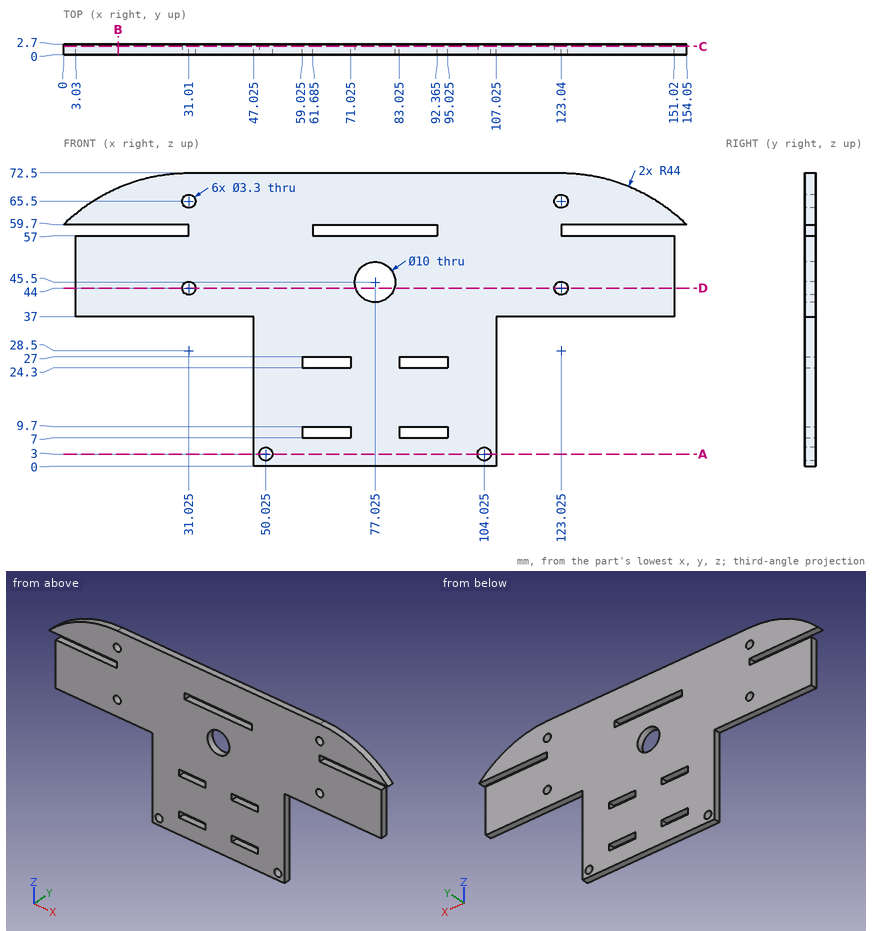
Check sheet for the drawn part. Datum: minimum x, y, z corner. Units: mm. Give positions to 0.01 mm unless a question says otherwise; leave off trailing zeros. Write each loop counter-clockwise with the first axis right and the second up, starting at its lowest first coordinate (ties: lowest second). Pieces come first, ordered by that corner, then holes. Notation, with made-up numbers: M 80,63.5 L 119,63.5 A18 ccw 119,81.5 Z; hole C 67.25,-14.5 d2. An arc over 180 degrees is marked long. One line per question, with ' | ' between items.
1. Cross-section at C-C (y = 2.1). Count the separate pieces of the cut face and the enclosed holes in it, plus the area to 3 significant figures.
Ans:
separate pieces: 1 | enclosed holes: 12 | area: 6,810 mm2
2. Scan lines: line 1 along Z through (x, y) = (70.5, 2.5); line 2 along X through (y, z) = (1.2, 3) (1 decimal); line 3 along X through (y, z) = (1.2, 44) (1 decimal). Record each from-to range of solid material in increasing order. Write a range as from..to.
Ans:
line 1: 0..7, 9.7..24.3, 27..57, 59.7..72.5 | line 2: 47..48.4, 51.7..102.4, 105.7..107 | line 3: 3..29.4, 32.7..72.3, 81.8..121.4, 124.7..151
3. Cross-section at D-D (z = 44). Enter the section's corners in (x, y) (1 decimal).
Ans:
outline: M 3,0 L 29.4,0 L 29.4,2.7 L 3,2.7 Z; M 32.7,0 L 72.3,0 L 72.3,2.7 L 32.7,2.7 Z; M 81.8,0 L 121.4,0 L 121.4,2.7 L 81.8,2.7 Z; M 124.7,0 L 151,0 L 151,2.7 L 124.7,2.7 Z
4. Gauge pin test, flat ends, axial feed: pin 1 (6 mm diameter, centred on x = 77.03, z = 45.5, fed in from -Y); pin 2 (1.4 mm diameter, centred on y = 1, z = 58, fed in from +X); pin 3 (1 mm diameter, centred on x = 131, y = 1.5, fed in from +Z); pin 4 (0.8 mm diameter, centred on y = 1, z = 42, fed in from +X). Record the tip position at first contact, or that the pin passes through.
Ans:
pin 1: through | pin 2: x = 123.04 | pin 3: z = 71.86 | pin 4: x = 151.02
5. Cross-section at B-B (x = 13.5). Enter the section's corners in (y, z).
Ans:
outline: M 0,37 L 2.7,37 L 2.7,57 L 0,57 Z; M 0,59.7 L 2.7,59.7 L 2.7,68.86 L 0,68.86 Z
6. Cross-section at A-A (z = 3). Enter the section's corners in (x, y) (1 decimal).
Ans:
outline: M 47,0 L 48.4,0 L 48.4,2.7 L 47,2.7 Z; M 51.7,0 L 102.4,0 L 102.4,2.7 L 51.7,2.7 Z; M 105.7,0 L 107,0 L 107,2.7 L 105.7,2.7 Z
